```python
from build123d import *

# Parameters (mm, degrees)
SKETCH1_W               = 63
SKETCH1_H               = 63
SKETCH1_W_2             = 56
SKETCH1_H_2             = 56
SKETCH1_W_3             = 12
SKETCH1_H_3             = 10
SKETCH1_R               = 1.55
BOSS_EXTRUDE1_DEPTH     = 2.5
SKETCH1_3_W             = 63
SKETCH1_3_H             = 63
SKETCH1_3_W_2           = 56
SKETCH1_3_H_2           = 56
BOSS_EXTRUDE2_DEPTH     = 10
SKETCH1_4_W             = 12
SKETCH1_4_H             = 10
SKETCH1_4_R             = 1.55
BOSS_EXTRUDE3_DEPTH     = 2
FILLET1_R               = 3
FILLET2_R               = 2
CHAMFER1_SIZE           = 1
CUT_EXTRUDE1_DEPTH      = 85.288196089
CUT_EXTRUDE1_DEPTH_BACK = 85.288196089
SKETCH2_R               = 1.5
FILLET3_R               = 0.5


with BuildPart() as part:
    # Sketch1 → Boss-Extrude1 (new body)
    # profile 1 of 6: a face of its own
    with BuildSketch(Plane.XY):
        with Locations((0, -40)):
            Rectangle(SKETCH1_W, SKETCH1_H)
        with Locations((0, -40)):
            Rectangle(SKETCH1_W_2, SKETCH1_H_2, mode=Mode.SUBTRACT)
    # profile 2 of 6: a face of its own
    with BuildSketch(Plane.XY):
        with Locations((0, -40)):
            Rectangle(SKETCH1_W_2, SKETCH1_H_2)
    # profile 3 of 6: a face of its own
    with BuildSketch(Plane.XY):
        with Locations((37.5, -13.5)):
            Rectangle(SKETCH1_W_3, SKETCH1_H_3)
        with Locations((38.5, -13.5)):
            Circle(SKETCH1_R, mode=Mode.SUBTRACT)
    # profile 4 of 6: a face of its own
    with BuildSketch(Plane.XY):
        with Locations((37.5, -66.5)):
            Rectangle(SKETCH1_W_3, SKETCH1_H_3)
        with Locations((38.5, -66.5)):
            Circle(SKETCH1_R, mode=Mode.SUBTRACT)
    # profile 5 of 6: a face of its own
    with BuildSketch(Plane.XY):
        with Locations((-37.5, -66.5)):
            Rectangle(SKETCH1_W_3, SKETCH1_H_3)
        with Locations((-38.5, -66.5)):
            Circle(SKETCH1_R, mode=Mode.SUBTRACT)
    # profile 6 of 6: a face of its own
    with BuildSketch(Plane.XY):
        with Locations((-37.5, -13.5)):
            Rectangle(SKETCH1_W_3, SKETCH1_H_3)
        with Locations((-38.5, -13.5)):
            Circle(SKETCH1_R, mode=Mode.SUBTRACT)
    extrude(amount=BOSS_EXTRUDE1_DEPTH)

    # Sketch1<3> → Boss-Extrude2 (add)
    with BuildSketch(Plane.XY):
        with Locations((0, -40)):
            Rectangle(SKETCH1_3_W, SKETCH1_3_H)
        with Locations((0, -40)):
            Rectangle(SKETCH1_3_W_2, SKETCH1_3_H_2, mode=Mode.SUBTRACT)
    extrude(amount=BOSS_EXTRUDE2_DEPTH)

    # Sketch1<4> → Boss-Extrude3 (add)
    # profile 1 of 4: a face of its own
    with BuildSketch(Plane.XY):
        with Locations((-37.5, -66.5)):
            Rectangle(SKETCH1_4_W, SKETCH1_4_H)
        with Locations((-38.5, -66.5)):
            Circle(SKETCH1_4_R, mode=Mode.SUBTRACT)
    # profile 2 of 4: a face of its own
    with BuildSketch(Plane.XY):
        with Locations((-37.5, -13.5)):
            Rectangle(SKETCH1_4_W, SKETCH1_4_H)
        with Locations((-38.5, -13.5)):
            Circle(SKETCH1_4_R, mode=Mode.SUBTRACT)
    # profile 3 of 4: a face of its own
    with BuildSketch(Plane.XY):
        with Locations((37.5, -13.5)):
            Rectangle(SKETCH1_4_W, SKETCH1_4_H)
        with Locations((38.5, -13.5)):
            Circle(SKETCH1_4_R, mode=Mode.SUBTRACT)
    # profile 4 of 4: a face of its own
    with BuildSketch(Plane.XY):
        with Locations((37.5, -66.5)):
            Rectangle(SKETCH1_4_W, SKETCH1_4_H)
        with Locations((38.5, -66.5)):
            Circle(SKETCH1_4_R, mode=Mode.SUBTRACT)
    extrude(amount=BOSS_EXTRUDE3_DEPTH)

    # Fillet1
    fillet1_edges = [part.edges().sort_by_distance(p)[0] for p in [
        (-31.5, -18.5, 1.25),
        (-43.5, -18.5, 1.25),
        (-43.5, -8.5, 1.25),
        (43.5, -8.5, 1.25),
        (43.5, -18.5, 1.25),
        (31.5, -18.5, 1.25),
        (31.5, -61.5, 1.25),
        (43.5, -61.5, 1.25),
        (43.5, -71.5, 1.25),
        (-43.5, -71.5, 1.25),
        (-43.5, -61.5, 1.25),
        (-31.5, -61.5, 1.25),
    ]]
    fillet(fillet1_edges, radius=FILLET1_R)

    # Fillet2
    fillet2_edges = [part.edges().sort_by_distance(p)[0] for p in [
        (-31.5, -71.5, 6.25),
        (31.5, -8.5, 6.25),
        (-31.5, -8.5, 6.25),
        (31.5, -71.5, 6.25),
    ]]
    fillet(fillet2_edges, radius=FILLET2_R)

    # Chamfer1
    chamfer1_edges = [part.edges().sort_by_distance(p)[0] for p in [
        (28, -40, 10),
        (0, -68, 10),
        (-28, -40, 10),
        (0, -12, 10),
    ]]
    chamfer(chamfer1_edges, length=CHAMFER1_SIZE)

    # Sketch2 → Cut-Extrude1 (cut, two sides: drawn at the far end of the back side and taken through both)
    with BuildSketch(Plane(origin=(0, 0, 0), x_dir=(-1, 0, 0), z_dir=(0, 0, -1)).offset(-CUT_EXTRUDE1_DEPTH_BACK)):
        with Locations((-21.5, -18.5)):
            Circle(SKETCH2_R)
        with Locations((-21.5, -61.5)):
            Circle(SKETCH2_R)
        with Locations((21.5, -61.5)):
            Circle(SKETCH2_R)
        with Locations((21.5, -18.5)):
            Circle(SKETCH2_R)
    extrude(amount=CUT_EXTRUDE1_DEPTH + CUT_EXTRUDE1_DEPTH_BACK, mode=Mode.SUBTRACT)

    # Fillet3
    fillet3_edges = [part.edges().sort_by_distance(p)[0] for p in [
        (23, -61.5, 0),
        (-20, -61.5, 0),
        (23, -18.5, 0),
        (-20, -18.5, 0),
    ]]
    fillet(fillet3_edges, radius=FILLET3_R)


solid = part.part
```
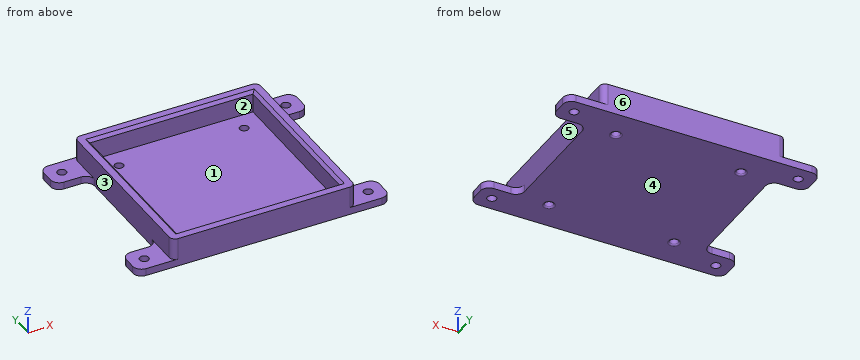
Geometry: final body of the model. Coordinates: model frame, mm. Face numbers are marked on the shaded views. A direction names the side the tool comes from. Coordinates: 2 decimals unless noted, no trailing zeros. Loops run counter-clockwise (first coordinate to the right, second up) from the corner with the lowest first, then second, coordinate; pieces in that order, holes last. Notation, with made-up numbers: M 13.5,-31 L 56.5,-31 A30 ccw 56.5,8 Z; hole C 4,-3.75 d3. An arc over 180 degrees is marked long. Put each result on its own line as item: value.
(1) Draft query along X for the marked faces 1, 2, 3 and 4. Return one class per face: pulls with the +X half, pulls with the -X half, needs draft (parallel to the pull), parting line crosses it, or undercut.
Answer sheet:
face 1: undercut
face 2: undercut
face 3: pulls with the -X half
face 4: needs draft
(2) Cut plane A-A on z = 4. Return the cut outline in (x, y), then the cut area to 3 significant figures.
Answer sheet:
outline: M -31.5,-69.5 A2 ccw -29.5,-71.5 L 29.5,-71.5 A2 ccw 31.5,-69.5 L 31.5,-10.5 A2 ccw 29.5,-8.5 L -29.5,-8.5 A2 ccw -31.5,-10.5 Z; hole M -28,-68 L 28,-68 L 28,-12 L -28,-12 Z
area: 830 mm^2
(3) Material intervals for probe 1 along X at (y, z) = (-66.5, 1.7); probe 2 along Y at (x, z) = (38.5, 0.9); probe 3 along Y at (x, z) = (-21.5, 0.9), sorted ascending.
Answer sheet:
probe 1: x = -43.5 to -40.05, -36.95 to 36.95, 40.05 to 43.5
probe 2: y = -71.5 to -68.05, -64.95 to -61.5, -18.5 to -15.05, -11.95 to -8.5
probe 3: y = -71.5 to -63, -60 to -20, -17 to -8.5
(4) Cut plane B-B on x = -38.5. Return the cut outline in (y, z).
Answer sheet:
outline: M -71.5,0 L -68.05,0 L -68.05,2.5 L -71.5,2.5 Z; M -64.95,0 L -61.5,0 L -61.5,2.5 L -64.95,2.5 Z; M -18.5,0 L -15.05,0 L -15.05,2.5 L -18.5,2.5 Z; M -11.95,0 L -8.5,0 L -8.5,2.5 L -11.95,2.5 Z
(5) Cut plane D-D on x = 27. Return the cut outline in (y, z).
Answer sheet:
outline: M -71.5,0 L -8.5,0 L -8.5,10 L -11,10 L -12,9 L -12,2.5 L -68,2.5 L -68,9 L -69,10 L -71.5,10 Z
(6) First-contact query: pin 1 (5 mm diameter, centred on x = 38.5, y = -66.5, fed in from +Z); pin 2 (3 mm diameter, centred on y = -38.5, z = 4.5, fed in from -X); pin 3 (2.5 mm diameter, centred on x = -21.5, y = -61.5, fed in from -Z); pin 4 (2 mm diameter, centred on x = 32, z = 8, fed in from -Y). Flat tips, straight axial feed; report the tip coordinate or a pass-through.
Answer sheet:
pin 1: stops at z = 2.5
pin 2: stops at x = -31.5
pin 3: passes through
pin 4: stops at y = -70.82
(7) Cut plane C-C on y = -66.5. Return the cut outline in (x, z), then the cut area to 4 significant figures.
Answer sheet:
outline: M -43.5,0 L -40.05,0 L -40.05,2.5 L -43.5,2.5 Z; M -36.95,0 L 36.95,0 L 36.95,2.5 L 31.5,2.5 L 31.5,10 L 29,10 L 28,9 L 28,2.5 L -28,2.5 L -28,9 L -29,10 L -31.5,10 L -31.5,2.5 L -36.95,2.5 Z; M 40.05,0 L 43.5,0 L 43.5,2.5 L 40.05,2.5 Z
area: 253.5 mm^2
(8) Access query for the marked faces 5 and 6. Directions: +Z, -Z, +X, -X, +Y, -Y. A direction counts if a zero-diameter tool reaches every point of the face in a straight line with its end or side. Return the directions, or none.
Answer sheet:
face 5: +Z, +X
face 6: +Z, -Z, +X, -X, +Y
